```python
from build123d import *

# Parameters (mm, degrees)
SKETCH1_W           = 30
SKETCH1_H           = 30
SKETCH1_W_2         = 27
SKETCH1_H_2         = 27
BOSS_EXTRUDE1_DEPTH = 250
SKETCH2_R           = 2.5
SKETCH2_R_2         = 3.1
CUT_EXTRUDE1_DEPTH  = 254.574446662
SKETCH3_R           = 2.2
CUT_EXTRUDE2_DEPTH  = 254.574446662


with BuildPart() as part:
    # Sketch1 → Boss-Extrude1 (new body)
    with BuildSketch(Plane.XY):
        with Locations((15, 15)):
            Rectangle(SKETCH1_W, SKETCH1_H)
        with Locations((15, 15)):
            Rectangle(SKETCH1_W_2, SKETCH1_H_2, mode=Mode.SUBTRACT)
    extrude(amount=BOSS_EXTRUDE1_DEPTH)

    # Sketch2 → Cut-Extrude1 (cut, through all)
    with BuildSketch(Plane(origin=(30, 0, 0), x_dir=(0, 0, -1), z_dir=(1, 0, 0))):
        with Locations((-15, 15)):
            Circle(SKETCH2_R)
        with Locations((-235, 15)):
            Circle(SKETCH2_R)
        with Locations((-175, 20)):
            Circle(SKETCH2_R_2)
        with BuildLine():
            Line((-142.5, 16.75), (-147.5, 16.75))
            ThreePointArc((-147.5, 16.75), (-149.25, 15), (-147.5, 13.25))
            Line((-147.5, 13.25), (-142.5, 13.25))
            ThreePointArc((-142.5, 13.25), (-140.75, 15), (-142.5, 16.75))
        make_face()
        with BuildLine():
            Line((-107.5, 16.75), (-102.5, 16.75))
            ThreePointArc((-102.5, 16.75), (-100.75, 15), (-102.5, 13.25))
            Line((-102.5, 13.25), (-107.5, 13.25))
            ThreePointArc((-107.5, 13.25), (-109.25, 15), (-107.5, 16.75))
        make_face()
        with BuildLine():
            Line((-125, 19.25), (-127.5, 19.25))
            ThreePointArc((-127.5, 19.25), (-131.75, 15), (-127.5, 10.75))
            Line((-127.5, 10.75), (-125, 10.75))
            Line((-125, 10.75), (-122.5, 10.75))
            ThreePointArc((-122.5, 10.75), (-118.25, 15), (-122.5, 19.25))
            Line((-122.5, 19.25), (-125, 19.25))
        make_face()
        with BuildLine():
            Line((-75, 23.1), (-85, 23.1))
            ThreePointArc((-85, 23.1), (-88.1, 20), (-85, 16.9))
            Line((-85, 16.9), (-75, 16.9))
            Line((-75, 16.9), (-65, 16.9))
            ThreePointArc((-65, 16.9), (-61.9, 20), (-65, 23.1))
            Line((-65, 23.1), (-75, 23.1))
        make_face()
    extrude(amount=-CUT_EXTRUDE1_DEPTH, mode=Mode.SUBTRACT)

    # Sketch3 → Cut-Extrude2 (cut, through all)
    with BuildSketch(Plane(origin=(0, 30, 0), x_dir=(1, 0, 0), z_dir=(0, 1, 0))):
        with Locations(Location((15, -25, 0), (0, 0, 270))):
            Circle(SKETCH3_R)
        with Locations(Location((15, -225, 0), (0, 0, 270))):
            Circle(SKETCH3_R)
    extrude(amount=-CUT_EXTRUDE2_DEPTH, mode=Mode.SUBTRACT)


solid = part.part
```
Read the model definition and answer for the solid it produces. Units are mm, in the model's axes. A direction names the side the tool comes from. Coordinates: 2 decimals unless noted, no trailing zeros. Write each loop counter-clockwise with the first axis right and the second up, starting at its lowest first coordinate (ties: lowest second). Pieces come first, ordered by that corner, then holes. Notation, with made-up numbers: (-5, 32) - (17, 32) arc R20 cw to (17, 71) - close; hole circle Ø5 at (-7, 49). An arc over 180 degrees is marked (long way). Answer as a JSON object with one key per item and string values. Group by question number.
1. The mould has two halves that part along Z. Classify faces 1 (the cylindrical face through (0.761, 15.751, 232.615)), 2 (the flat face through (15, 1.5, 123)), 3 (the flat face through (14, 1, 0)), 4 (the cylindrical face through (29.26, 20.931, 172.043)): +Z half, -Z half, draft (parallel to the pull), parting line (faces both ways), or undercut.
2. A cutting plane is placed at D-D (z = 15). Determine the outline of the cut face in (x, y).
3. A cutting plane is placed at B-B (z = 50). Determine the outline of the cut face in (x, y), plus the area to 3 significant figures.
4. A cutting plane is placed at A-A (x = 23). Determine the outline of the cut face in (y, z).
5. Consider L1, parallel to Y at x = 6.5, z = 229; L2, parallel to X at y = 29.15, z = 225. Determine where each line is inside the solid, lowest interval first. Write a range as [from, to].
6. Each of these flat-tipped pins is pushed along its axis until it touches: P1, Ø1.2, axis at x = 1, z = 146, coming from the -Y side; P2, Ø4, axis at x = 15, z = 25, coming from the +Y side. Where does it stop, or does it pass through?
7. Which of the six approach directions +Z, -Z, +X, -X, +Y, -Y give full straight-line access (tool end or side, diameter ignored) to faces 5 (the flat face through (28.5, 9, 123)), 6 (the cylindrical face through (0.76, 15.09, 131.75)), 7 (the flat face through (30, 8, 123))?
Worked out:
{
 "1": {"face 1": "undercut", "face 2": "draft", "face 3": "-Z half", "face 4": "undercut"},
 "2": {"outline": "(0, 0) - (30, 0) - (30, 12.5) - (28.5, 12.5) - (28.5, 1.5) - (1.5, 1.5) - (1.5, 12.5) - (0, 12.5) - close; (0, 17.5) - (1.5, 17.5) - (1.5, 28.5) - (28.5, 28.5) - (28.5, 17.5) - (30, 17.5) - (30, 30) - (0, 30) - close"},
 "3": {"outline": "(0, 0) - (30, 0) - (30, 30) - (0, 30) - close; hole (1.5, 1.5) - (28.5, 1.5) - (28.5, 28.5) - (1.5, 28.5) - close", "area": "171 mm²"},
 "4": {"outline": "(0, 0) - (1.5, 0) - (1.5, 250) - (0, 250) - close; (28.5, 0) - (30, 0) - (30, 250) - (28.5, 250) - close"},
 "5": {"L1": "y = [0, 1.5], [28.5, 30]", "L2": "x = [0, 12.8], [17.2, 30]"},
 "6": {"P1": "stops at y = 0", "P2": "passes through"},
 "7": {"face 5": "+Z, -Z", "face 6": "+X, -X", "face 7": "+Z, -Z, +X, +Y, -Y"}
}
